from build123d import *

# Parameters (mm, degrees)
F0_W           = 1371.6
F0_H           = 76.2
F1_DEPTH       = 63.5
F2_D           = 8.2042
F2_CBORE_D     = 20.6375
F2_CBORE_DEPTH = 12.7


with BuildPart() as f1:
    # F0 (on Front) → F1 (new body)
    with BuildSketch(Plane.XZ):
        Rectangle(F0_W, F0_H)
    extrude(amount=-F1_DEPTH)

    # F2 (through all)
    with Locations(Plane.XZ):
        with Locations((-660.4, 0), (-330.2, 0), (0, 0), (330.2, 0), (660.4, 0)):
            CounterBoreHole(F2_D / 2, F2_CBORE_D / 2, F2_CBORE_DEPTH)


solid = f1.part
CAD build for the part. Positions are in the model's coordinates, mm. A direction names the side the tool comes from. Round coordinates to 2 decimals unless told otherwise and drop trailing zeros. Use a Markdown table: item, result. Add a question column.
1. 3-axis set-ups, long thin cutter, end or side, ignore diameter. For faces 4 (the face through (-330.3, 12.7, -4.4)), 5 (the face through (-10, 31, -38.1)): which of +Z, -Z, +X, -X, +Y, -Y reach the whole face in a straight line?
2. Pull direction Z, two halves, no side cores. Call faces 1 (the face through (-10, 0, 9)), 2 (the face through (-10, 31, 38.1)), 3 (the face through (335, 12.7, 0)): released by +Z, released by -Z, zero draft, split by the parting line, or undercut.
3. Drill centre lines: probe 1 along Z at (x, y) = (0, 6.5); probe 2 along Z at (x, y) = (330.2, 44.5). Where is each one in solid material? Low to high.
4. Flat gauge pin, fed straight in: P1, Ø10.5, axis at x = -665, z = 2, coming from the -Y side. Where does the tip first touch, or does it go through?
Reply:
| question | item | result |
|---|---|---|
| 1 | face 4 | -Y |
| 1 | face 5 | -Z, +X, -X, +Y, -Y |
| 2 | face 1 | zero draft |
| 2 | face 2 | released by +Z |
| 2 | face 3 | undercut |
| 3 | probe 1 | z = -38.1 to -10.32, 10.32 to 38.1 |
| 3 | probe 2 | z = -38.1 to -4.1, 4.1 to 38.1 |
| 4 | P1 | stops at y = 12.7 |
